The model under review builds one solid part; all positions refer to its coordinate system, in mm. A direction names the side the tool comes from. Round coordinates to 2 decimals unless told otherwise and drop trailing zeros. Order: outer loops, then holes, each group sorted by start corner. A loop starts at its lowest first (then second) coordinate and runs counter-clockwise, first axis right, second up. Notation, with made-up numbers: M -27.75,62.25 L 25.25,62.25 A32 cw 25.25,98.25 Z; hole C 75.5,85 d4. An arc over 180 degrees is marked long. One line per item, written item: value. Start each with the question number.
from build123d import *

# Parameters (mm, degrees)
SALIENTE_EXTRUIR1_DEPTH = 25.4
CROQUIS2_W              = 30
CROQUIS2_H              = 25.4
SALIENTE_EXTRUIR2_DEPTH = 1.5
CROQUIS4_R              = 2.5
CORTAR_EXTRUIR1_DEPTH   = 10


with BuildPart() as part:
    # Croquis1 → Saliente-Extruir1 (new body)
    with BuildSketch(Plane(origin=(0, 0, 0), x_dir=(1, 0, 0), z_dir=(0, 1, 0))):
        with BuildLine():
            Line((-58.5, 0), (-57, 0))
            ThreePointArc((-57, 0), (0, 57), (57, 0))
            Line((57, 0), (58.5, 0))
            ThreePointArc((58.5, 0), (0, 58.5), (-58.5, 0))
        make_face()
    extrude(amount=SALIENTE_EXTRUIR1_DEPTH)

    # Croquis2 → Saliente-Extruir2 (add)
    with BuildSketch(Plane.XY):
        with Locations((72, 12.7)):
            Rectangle(CROQUIS2_W, CROQUIS2_H)
        with Locations((-72, 12.7)):
            Rectangle(CROQUIS2_W, CROQUIS2_H)
    extrude(amount=-SALIENTE_EXTRUIR2_DEPTH)

    # Croquis4 → Cortar-Extruir1 (cut)
    with BuildSketch(Plane(origin=(0, 0, -1.5), x_dir=(-1, 0, 0), z_dir=(0, 0, -1))):
        with Locations((75.49, 13.164314045)):
            Circle(CROQUIS4_R)
        with Locations((-75.49, 13.164314045)):
            Circle(CROQUIS4_R)
    extrude(amount=-CORTAR_EXTRUIR1_DEPTH, mode=Mode.SUBTRACT)


solid = part.part
Item 1: Consider section A-A, the plane x = -75.49. Give the boundary of the cut face in (y, z), then the cut area to 3 significant figures.
Item 2: Consider section D-D, the plane x = 37. Give the boundary of the cut face in (y, z), then the cut area to 3 significant figures.
Item 3: The part is to be moulded in two halves that separate along Y. For faces 3 (the cylindrical face through (-72.992, 13.274, -0.76)), 4 (the cylindrical face through (73.1, 13.9, -0.8)), 5 (the flat face through (31.8, 25.4, -48.9)), 6 (the flat face through (-73, 10, -1.5)), say which applies: pulls with the +Y half, pulls with the -Y half, needs draft (parallel to the pull), parting line crosses it, or undercut.
Item 4: Clearance check with flat-ended pins moving along their axes: P1, Ø2, axis at y = 6, z = -32, coming from the +X side; P2, Ø12.5, axis at x = -72.5, y = 10.5, coming from the -Z side; P3, Ø12, axis at x = 46, y = 7, coming from the +Z side; P4, Ø4.5, axis at x = -75.49, y = 13.16, coming from the -Z side. State where each tip first meets the part, or that it passes through.
Item 5: Wall thickness on L1, parallel to Y at x = -75.49, z = -0.6; L2, parallel to X at y = 2.75, z = -15; L3, parallel to X at y = 13.5, z = -16: over which ranges is each line inside the solid? List them lowest first.
Item 6: Consider section B-B, the plane z = -7. Give the boundary of the cut face in (x, y).
Item 7: Consider section C-C, the plane y = 1.75. Give the boundary of the cut face in (x, z), then the cut area to 3 significant figures.
Item 8: Machinability: for faces 1 (the flat face through (31.8, 0, -48.9)), 2 (the flat face through (72.5, 12.9, -1.5)), which of the approach directions +Z, -Z, +X, -X, +Y, -Y give a long, thin tool a straight path to every point of the face, cutting with its end or side? Answer none if there is none.
Computed:
1. outline: M 0,-1.5 L 10.66,-1.5 L 10.66,0 L 0,0 Z; M 15.66,-1.5 L 25.4,-1.5 L 25.4,0 L 15.66,0 Z
1. area: 30.6 mm^2
2. outline: M 0,-45.31 L 25.4,-45.31 L 25.4,-43.36 L 0,-43.36 Z
2. area: 49.6 mm^2
3. face 3: undercut
3. face 4: undercut
3. face 5: pulls with the +Y half
3. face 6: needs draft
4. P1: stops at x = 49.61
4. P2: stops at z = -1.5
4. P3: stops at z = -23.35
4. P4: passes through
5. L1: y = 0 to 10.66, 15.66 to 25.4
5. L2: x = -56.54 to -54.99, 54.99 to 56.54
5. L3: x = -56.27 to -54.71, 54.71 to 56.27
6. outline: M -58.08,0 L -56.57,0 L -56.57,25.4 L -58.08,25.4 Z; M 56.57,0 L 58.08,0 L 58.08,25.4 L 56.57,25.4 Z
7. outline: M -87,-1.5 L -58.48,-1.5 A58.5 ccw 58.48,-1.5 L 87,-1.5 L 87,0 L 57,0 A57 cw -57,0 L -87,0 Z
7. area: 358 mm^2
8. face 1: +Z, -Z, +X, -X, -Y
8. face 2: -Z, +X, +Y, -Y
